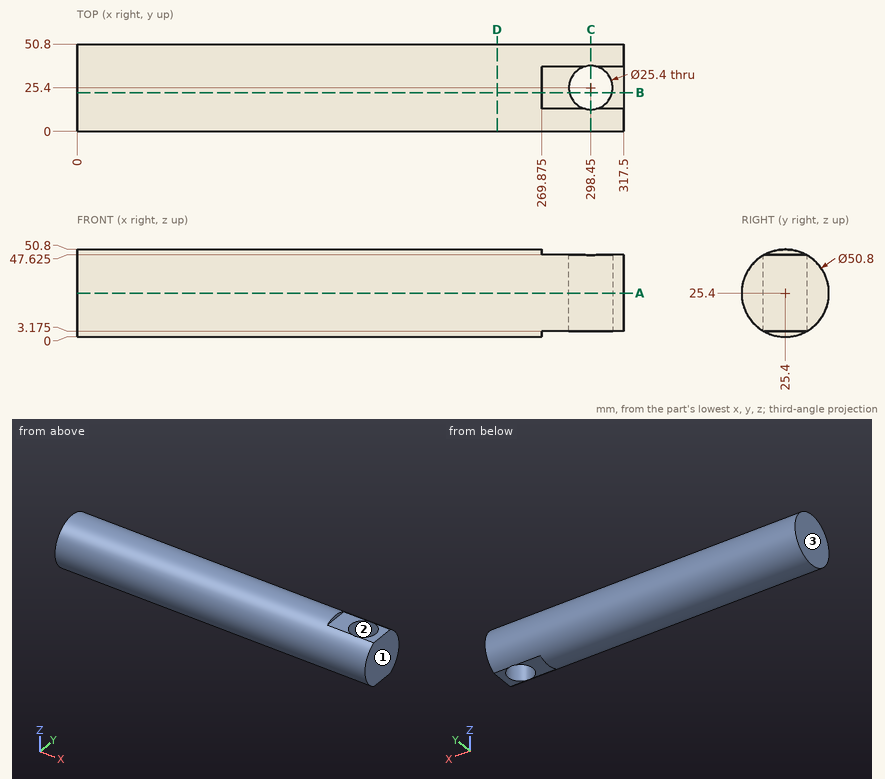
For this review, use the dimensioned drawing (mm, ordinates from the lowest corner) and the shaded views. Give positions to 0.01 mm unless a question says otherwise; leave off trailing zeros. Order: outer loops, then holes, each group sorted by start corner. A loop starts at its lowest first (then second) coordinate and runs counter-clockwise, first axis right, second up. Notation, with made-up numbers: (8, -13) - (46, -13) arc R15 ccw to (46, -4) - close; hole circle Ø8 at (63, 73). An arc over 180 degrees is marked (long way). Use a Markdown table: item, result. Add a question column.
(1) Clearance check with flat-ended pins moving along their axes: P1, Ø2, axis at x = 164, y = 13.5, coming from the -Z side; P2, Ø8, axis at x = 256, y = 6, coming from the +Z side; P3, Ø8, axis at x = 313.5, y = 20, coming from the +Z side (3 decimals). State where each tip first meets the part, or that it passes through.
(2) Mouldability with a two-part tool opening along X and no side actions: class the marked faces 1, 2 and 3 as +X half, -X half, draft (parallel to the pull), parting line (faces both ways), or undercut.
(3) Wall thickness on probe 1 along Y at (x, z) = (298.45, 26); probe 2 along X at (y, z) = (25, 35); probe 3 along X at (y, z) = (22, 14): over which ranges is each line inside the solid? List them lowest first. Write a range as [from, to].
(4) Add section D-D on x = 244. Give the boundary of the cut face in (y, z), then the cut area to 3 significant figures.
(5) Add section B-B on y = 22.5. Give the boundary of the cut face in (x, z) (3 decimals).
(6) Add section C-C on x = 298.45. Give the boundary of the cut face in (y, z).
(7) Add section A-A on z = 25.4. Give the boundary of the cut face in (x, y).
Report:
| question | item | result |
|---|---|---|
| 1 | P1 | stops at z = 2.46 |
| 1 | P2 | stops at z = 45.6 |
| 1 | P3 | stops at z = 47.625 |
| 2 | face 1 | +X half |
| 2 | face 2 | undercut |
| 2 | face 3 | -X half |
| 3 | probe 1 | y = [0.01, 12.7], [38.1, 50.79] |
| 3 | probe 2 | x = [0, 285.76], [311.14, 317.5] |
| 3 | probe 3 | x = [0, 286.21], [310.69, 317.5] |
| 4 | outline | circle Ø50.8 at (25.4, 25.4) |
| 4 | area | 2,030 mm² |
| 5 | outline | (0, 0.166) - (269.875, 0.166) - (269.875, 3.175) - (286.086, 3.175) - (286.086, 47.625) - (269.875, 47.625) - (269.875, 50.634) - (0, 50.634) - close; (310.814, 3.175) - (317.5, 3.175) - (317.5, 47.625) - (310.814, 47.625) - close |
| 6 | outline | (12.7, 3.4) - (12.7, 47.4) arc R25.4 ccw to start; (38.1, 3.4) arc R25.4 ccw to (38.1, 47.4) - close |
| 7 | outline | (0, 0) - (317.5, 0) - (317.5, 50.8) - (0, 50.8) - close; hole circle Ø25.4 at (298.45, 25.4) |
